Verification items for the finished model (mm, model axes). Round coordinates to 2 decimals unless told otherwise and drop trailing zeros. Write each loop counter-clockwise with the first axis right and the second up, starting at its lowest first coordinate (ties: lowest second). Pieces come first, ordered by that corner, then holes. Notation, with made-up numbers: (32.5, 86.25) - (91.5, 86.25) arc R13 ccw to (91.5, 100.25) - close; hole circle Ø10 at (54.5, 23). An arc over 180 degrees is marked (long way). Answer as a JSON object with one key per item and string values. Group by question number.
1) Section check A-A (y = 0). Enter the section's corners in (x, z) (3 decimals), then the cut area to 3 significant figures.
2) Section check C-C (z = 16.5). Enter the section's corners in (x, y).
3) Mould release check, pull along X, two halves, no side actions. Record for faces 1 (the cylindrical face through (6.883, 30.995, 16.958)), 2 (the flat face through (0, 0, 26.035)), 3 (the cylindrical face through (-2.54, -3.984, 30.864)), 4 (the flat face through (0, 6, 35.56)): +X half, -X half, draft (parallel to the pull), parting line (faces both ways), or undercut.
4) Thickness scan on line 1 (Z direction, x = 1.5, y = 0) (3 decimals); line 2 (X direction, y = 0, z = 28); line 3 (Y direction, x = -0.5, z = -14). Record the ranges inside material, lowest first.
5) Section check D-D (z = -22). Enter the section's corners in (x, y), then the cut area to 3 significant figures.
6) Go/stop test with flat-tipped pins: pin 1 Ø2 at (x, z) = (20.5, 23.5) entering from -Y; pin 2 Ø2 at (x, y) = (-16, 5) entering from -Z; pin 3 Ø6 at (y, z) = (-13, 28) entering from +X. Record where each tip stops, or that it passes through.
```python
from build123d import *

# Parameters (mm, degrees)
F3_R = 5.08
F5_R = 5.08


# Not quite as in the source:
# - a feature names something its author has since deleted; it is built from what else it names


with BuildPart() as f1:
    # F0 (on Front) → F1 (revolve)
    with BuildSketch(Plane.XZ):
        with BuildLine():
            Line((0, -5.842), (0, 0))
            Line((0, 0), (0, 3.81))
            Line((0, 3.81), (0, 16.51))
            Line((0, 16.51), (0, 26.035))
            Line((0, 26.035), (-4.7244, 26.035))
            Line((-4.7244, 26.035), (-4.7244, 35.56))
            Line((-4.7244, 35.56), (-7.2644, 35.56))
            Line((-7.2644, 35.56), (-31.75, 35.56))
            Line((-31.75, 35.56), (-31.75, 3.81))
            ThreePointArc((-31.75, 3.81), (-24.2400753332, -16.6956394155), (-5.2629922621, -27.5007555394))
            Line((-5.2629922621, -27.5007555394), (-1.6002, -27.8064487898))
            Line((-1.6002, -27.8064487898), (-1.6002, -5.842))
            Line((-1.6002, -5.842), (0, -5.842))
        make_face()
    revolve(axis=Axis((0, 0, 3.81), (0, 0, 1)))

    # F5
    f5_edges = [f1.edges().sort_by_distance(p)[0] for p in [
        (31.75, 0, 35.56),
    ]]
    fillet(f5_edges, radius=F5_R)


with BuildPart() as f2:
    # F0 (on Front) → F2 (revolve)
    with BuildSketch(Plane.XZ):
        with BuildLine():
            Line((0, -5.842), (0, 0))
            Line((0, 0), (0, 3.81))
            Line((0, 3.81), (0, 16.51))
            Line((0, 16.51), (0, 26.035))
            Line((0, 26.035), (-4.7244, 26.035))
            Line((-4.7244, 26.035), (-4.7244, 35.56))
            Line((-4.7244, 35.56), (-7.2644, 35.56))
            Line((-7.2644, 35.56), (-31.75, 35.56))
            Line((-31.75, 35.56), (-31.75, 3.81))
            ThreePointArc((-31.75, 3.81), (-24.2400753332, -16.6956394155), (-5.2629922621, -27.5007555394))
            Line((-5.2629922621, -27.5007555394), (-1.6002, -27.8064487898))
            Line((-1.6002, -27.8064487898), (-1.6002, -5.842))
            Line((-1.6002, -5.842), (0, -5.842))
        make_face()
    revolve(axis=Axis((0, 0, 3.81), (0, 0, 1)))

    # F3
    f3_edges = [f2.edges().sort_by_distance(p)[0] for p in [
        (31.75, 0, 35.56),
    ]]
    fillet(f3_edges, radius=F3_R)


solid = f1.part
```
Returned:
{
 "1": {"outline": "(-31.75, 3.81) arc R31.75 ccw to (-5.263, -27.501) - (-1.6, -27.806) - (-1.6, -5.842) - (1.6, -5.842) - (1.6, -27.806) - (5.263, -27.501) arc R31.75 ccw to (31.75, 3.81) - (31.75, 30.48) arc R5.08 ccw to (26.67, 35.56) - (4.724, 35.56) - (4.724, 26.035) - (-4.724, 26.035) - (-4.724, 35.56) - (-26.67, 35.56) arc R5.08 ccw to (-31.75, 30.48) - close", "area": "3,430 mm2"},
 "2": {"outline": "circle Ø63.5 at (0, 0)"},
 "3": {"face 1": "parting line", "face 2": "undercut", "face 3": "undercut", "face 4": "draft"},
 "4": {"line 1": "-5.842 to 26.035", "line 2": "-31.75 to -4.72, 4.72 to 31.75", "line 3": "-26.28 to -1.52, 1.52 to 26.28"},
 "5": {"outline": "circle Ø36.98 at (0, 0); hole circle Ø3.2 at (0, 0)", "area": "1,070 mm2"},
 "6": {"pin 1": "y = -25.06", "pin 2": "z = -23.75", "pin 3": "x = 30.13"}
}
